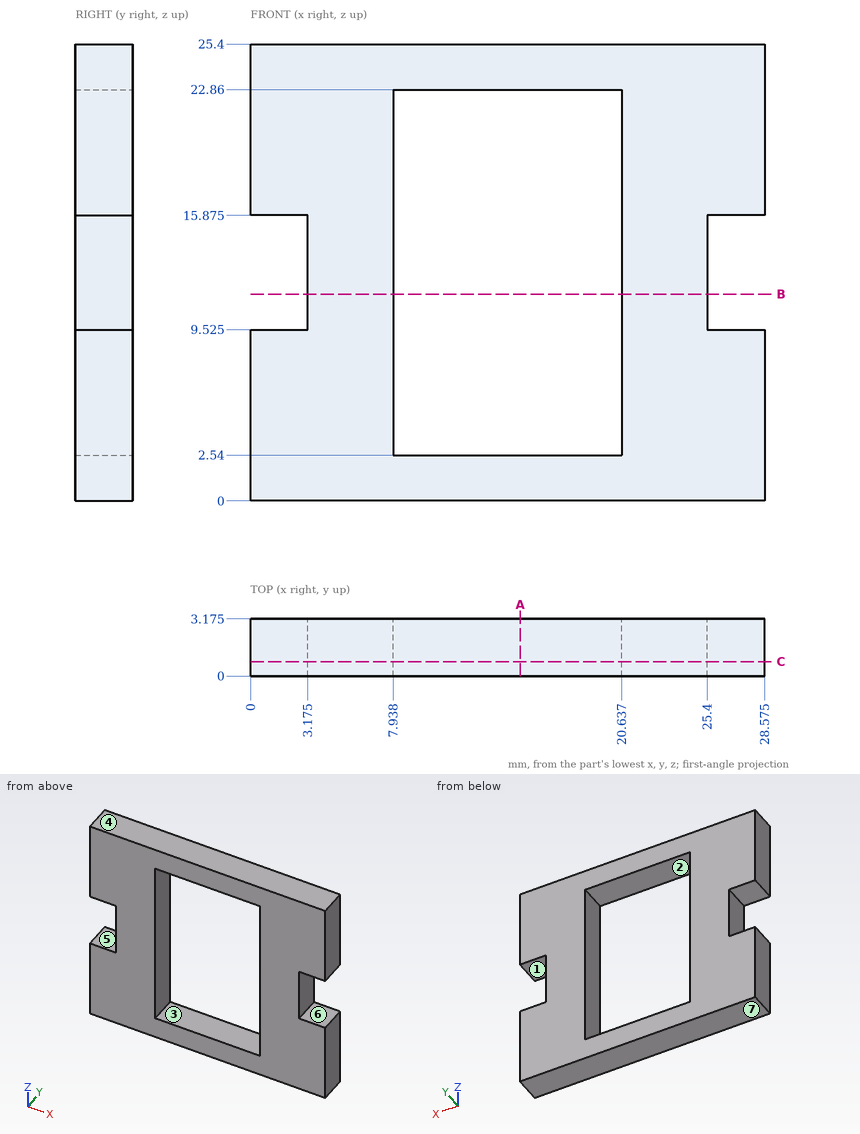
Job drawing, mm, ordinate dimensions from the low corner. One solid piece. A direction names the side the tool comes from. Round coordinates to 2 decimals unless told otherwise and drop trailing zeros. Write each loop counter-clockwise with the first axis right and the second up, starting at its lowest first coordinate (ties: lowest second). Pieces come first, ordered by that corner, then holes. Notation, with made-up numbers: M 18.5,68 L 26.5,68 A14 ccw 26.5,89 Z; hole C 76,-17 d11. An arc over 180 degrees is marked long. Return JSON: item names as keys, results as strings. Group by question number.
(1) Saw through at C-C on y = 0.8. Write the cut outline in (x, z) (1 decimal).
(2) Which spindle directions (+Z, -Z, +X, -X, +Y, -Y) get a long thin tool onto all of the face, cutting with end or side? Do the marked faces 3, 4, 5, 6 and 7. Say none if no direction does.
(3) Drill centre lines: probe 1 along Z at (x, y) = (16.5, 3.05); probe 2 along X at (y, z) = (2.4, 21.75) (1 decimal); probe 3 along Z at (x, y) = (25.5, 1.7) (1 decimal). Where is each one in solid material? Low to high.
(4) Pin check, flat tips, straight feed: pin 1 Ø1 at (x, y) = (20.5, 3) entering from -Z; pin 2 Ø1 at (y, z) = (2, 12) entering from +X. Stop position of each tip, or through.
(5) Saw through at A-A on x = 15. Write the cut outline in (y, z) (1 decimal).
(6) Saw through at B-B on z = 11.5. Write the cut outline in (x, y) (1 decimal).
(7) Two-plate mould, pull along X, no slides. Class the marked faces 1 and 2: +X half, -X half, draft (parallel to the pull), parting line (faces both ways), or undercut.
Returned:
{
 "1": {"outline": "M 0,0 L 28.6,0 L 28.6,9.5 L 25.4,9.5 L 25.4,15.9 L 28.6,15.9 L 28.6,25.4 L 0,25.4 L 0,15.9 L 3.2,15.9 L 3.2,9.5 L 0,9.5 Z; hole M 7.9,2.5 L 20.6,2.5 L 20.6,22.9 L 7.9,22.9 Z"},
 "2": {"face 3": "+Y, -Y", "face 4": "+Z, +X, -X, +Y, -Y", "face 5": "-X, +Y, -Y", "face 6": "+X, +Y, -Y", "face 7": "-Z, +X, -X, +Y, -Y"},
 "3": {"probe 1": "0 to 2.54, 22.86 to 25.4", "probe 2": "0 to 7.9, 20.6 to 28.6", "probe 3": "0 to 9.5, 15.9 to 25.4"},
 "4": {"pin 1": "z = 0", "pin 2": "x = 25.4"},
 "5": {"outline": "M 0,0 L 3.2,0 L 3.2,2.5 L 0,2.5 Z; M 0,22.9 L 3.2,22.9 L 3.2,25.4 L 0,25.4 Z"},
 "6": {"outline": "M 3.2,0 L 7.9,0 L 7.9,3.2 L 3.2,3.2 Z; M 20.6,0 L 25.4,0 L 25.4,3.2 L 20.6,3.2 Z"},
 "7": {"face 1": "draft", "face 2": "undercut"}
}
